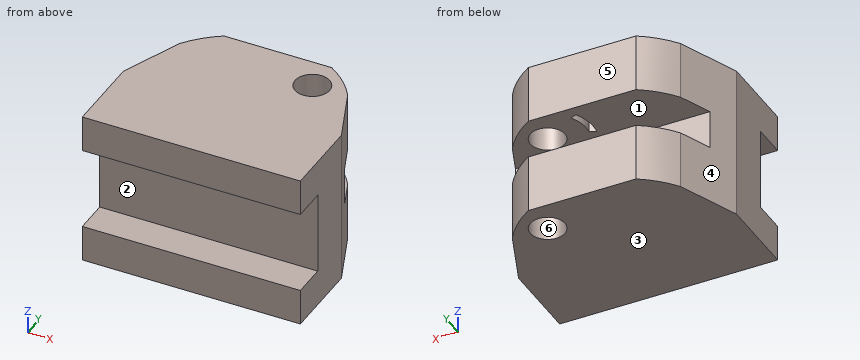
from build123d import *

# Parameters (mm, degrees)
SKETCH1_W           = 64
SKETCH1_H           = 33
BOSS_EXTRUDE2_DEPTH = 90
SKETCH5_W           = 34
SKETCH5_H           = 14
CUT_EXTRUDE1_DEPTH  = 91
SKETCH7_W           = 90
SKETCH7_H           = 64
BOSS_EXTRUDE3_DEPTH = 37
SKETCH9_W           = 16
SKETCH9_H           = 25
CUT_EXTRUDE2_DEPTH  = 91
CUT_EXTRUDE3_DEPTH  = 65
CUT_EXTRUDE4_DEPTH  = 65
SKETCH12_R          = 4.563258517
CUT_EXTRUDE5_DEPTH  = 65
SKETCH13_R          = 3.396180785
CUT_EXTRUDE7_DEPTH  = 4
SKETCH14_R          = 7.131807436
CUT_EXTRUDE8_DEPTH  = 65
CUT_EXTRUDE9_START  = -17
CUT_EXTRUDE9_DEPTH  = 30


with BuildPart() as part:
    # Sketch1 → Boss-Extrude2 (new body)
    with BuildSketch(Plane(origin=(0, 0, 0), x_dir=(0, 0, -1), z_dir=(1, 0, 0))):
        Rectangle(SKETCH1_W, SKETCH1_H)
    extrude(amount=BOSS_EXTRUDE2_DEPTH)

    # Sketch5 → Cut-Extrude1 (cut, through all)
    with BuildSketch(Plane.ZY):
        with Locations((0, -9.5)):
            Rectangle(SKETCH5_W, SKETCH5_H)
    extrude(amount=-CUT_EXTRUDE1_DEPTH, mode=Mode.SUBTRACT)

    # Sketch7 → Boss-Extrude3 (add)
    with BuildSketch(Plane(origin=(0, 16.5, 0), x_dir=(1, 0, 0), z_dir=(0, 1, 0))):
        with Locations((45, 0)):
            Rectangle(SKETCH7_W, SKETCH7_H)
    extrude(amount=BOSS_EXTRUDE3_DEPTH)

    # Sketch9 → Cut-Extrude2 (cut, through all)
    with BuildSketch(Plane.ZY):
        with Locations((0, 41)):
            Rectangle(SKETCH9_W, SKETCH9_H)
    extrude(amount=-CUT_EXTRUDE2_DEPTH, mode=Mode.SUBTRACT)

    # Sketch10 → Cut-Extrude3 (cut, through all)
    with BuildSketch(Plane.XY.offset(32)):
        Polygon((0, 16.5), (15, 53.5), (0, 53.5), align=None)
        Polygon((90, 53.5), (90, 16.5), (75, 53.5), align=None)
    extrude(amount=-CUT_EXTRUDE3_DEPTH, mode=Mode.SUBTRACT)

    # Sketch11 → Cut-Extrude4 (cut, through all)
    with BuildSketch(Plane.XY.offset(32)):
        with BuildLine():
            Line((22.559269827, 53.5), (15, 53.5))
            Line((15, 53.5), (10.196218084, 41.650671273))
            ThreePointArc((10.196218084, 41.650671273), (15.770987206, 48.208398087), (22.559269827, 53.5))
        make_face()
        with BuildLine():
            Line((80.252850536, 40.542968678), (75, 53.5))
            Line((75, 53.5), (66.982723611, 53.5))
            ThreePointArc((66.982723611, 53.5), (74.341930784, 47.763126364), (80.252850536, 40.542968678))
        make_face()
    extrude(amount=-CUT_EXTRUDE4_DEPTH, mode=Mode.SUBTRACT)

    # Sketch12 → Cut-Extrude5 (cut, through all)
    with BuildSketch(Plane(origin=(0, 0, -32), x_dir=(-1, 0, 0), z_dir=(0, 0, -1))):
        with Locations((-65.890311292, 40.12330388)):
            Circle(SKETCH12_R)
    extrude(amount=-CUT_EXTRUDE5_DEPTH, mode=Mode.SUBTRACT)

    # Sketch13 → Cut-Extrude7 (cut)
    with BuildSketch(Plane(origin=(0, 28.5, 0), x_dir=(1, 0, 0), z_dir=(0, 1, 0))):
        with Locations((18.559847102, 1.303256126)):
            Circle(SKETCH13_R)
    extrude(amount=-CUT_EXTRUDE7_DEPTH, mode=Mode.SUBTRACT)

    # Sketch14 → Cut-Extrude8 (cut, through all)
    with BuildSketch(Plane.XY.offset(32)):
        with Locations((65.890311292, 40.12330388)):
            Circle(SKETCH14_R)
    extrude(amount=-CUT_EXTRUDE8_DEPTH, mode=Mode.SUBTRACT)

    # Sketch15 → Cut-Extrude9 (cut)
    with BuildSketch(Plane.XY.offset(32).offset(CUT_EXTRUDE9_START)):
        with BuildLine():
            Line((52.144239181, 48.178611287), (49.568050992, 49.212876474))
            ThreePointArc((49.568050992, 49.212876474), (47.410527131, 42.86813331), (47.630804887, 36.170211787))
            Line((47.630804887, 36.170211787), (50.191024462, 37.407632885))
            ThreePointArc((50.191024462, 37.407632885), (50.21355191, 42.966135424), (52.144239181, 48.178611287))
        make_face()
    extrude(amount=-CUT_EXTRUDE9_DEPTH, mode=Mode.SUBTRACT)


solid = part.part
Can you work these out from the model? Positions are in its coordinate system, mm. Face numbers are marked on the shaded views. A direction names the side the tool comes from. Round coordinates to 2 decimals unless told otherwise and drop trailing zeros. Loops run counter-clockwise (first coordinate to the right, second up) from the corner with the lowest first, then second, coordinate; pieces in that order, holes last. Notation, with made-up numbers: (44, -4.5) - (69, -4.5) arc R17 cw to (69, 25.5) - close; hole circle Ø4 at (68, -30.5). An arc over 180 degrees is marked (long way). Write item = value, one per line. Start each with the question number.
(1) If we section it at A-A (y = -10.5): Please give me the cut outline in (x, z).
(2) If we section it at D-D (x = 63): Please give me the cut outline in (y, z), and give its area (3 significant figures).
(3) For the marked faces 1, 2 and 3, which set-ups out of +Z, -Z, +X, -X, +Y, -Y let a thin tool reach every point of the face, with its end or its side?
(4) If we mould it in two halves opening along X, with no side actions, what happens to the marked faces 4, 5 and 6? For each: released by +X, released by -X, zero draft, split by the parting line, or undercut.
(5) If I drill on probe 1 along Z at (x, y) = (81.5, -13); probe 2 along Y at (x, z) = (42.5, -0.5); probe 3 along Z at (x, y) = (45.5, 47), over which ranges is the centre line in solid material (lowest first)? Write a range as [from, to].
(6) If we section it at B-B (x = 54): Please give me the cut outline in (y, z).
(7) For P1, Ø4, axis at x = 54.5, z = -3.5, coming from the -Y side; P2, Ø7.5, axis at x = 17, z = 0, coming from the +Y side; P3, Ø13, axis at x = 65.89, y = 40.12, coming from the -Z side; P4, Ø4, axis at x = 18.56, z = -1.3, coming from the +Y side, each with a flat end and sliding along its axis, tell me the tip position at first contact or that it passes through.
(8) If we section it at C-C (z = -18.5): Please give me the cut outline in (x, y).
Ans:
q1.outline = (0, -32) - (90, -32) - (90, -17) - (0, -17) - close; (0, 17) - (90, 17) - (90, 32) - (0, 32) - close
q2.outline = (-16.5, -32) - (33.6, -32) - (33.6, -8) - (28.5, -8) - (28.5, 8) - (33.6, 8) - (33.6, 32) - (-16.5, 32) - (-16.5, 17) - (-2.5, 17) - (-2.5, -17) - (-16.5, -17) - close; (46.64, -32) - (53.5, -32) - (53.5, -8) - (46.64, -8) - close; (46.64, 8) - (53.5, 8) - (53.5, 32) - (46.64, 32) - close
q2.area = 2,980 mm²
q3.face_1 = +X, -X, +Y
q3.face_2 = +X, -X, -Y
q3.face_3 = -Z, +X, -X, +Y, -Y
q4.face_4 = released by -X
q4.face_5 = zero draft
q4.face_6 = undercut
q5.probe_1 = [-32, -17], [17, 32]
q5.probe_2 = [-2.5, 28.5]
q5.probe_3 = [-32, -8], [8, 32]
q6.outline = (-16.5, -32) - (53.5, -32) - (53.5, -8) - (28.5, -8) - (28.5, 8) - (53.5, 8) - (53.5, 32) - (-16.5, 32) - (-16.5, 17) - (-2.5, 17) - (-2.5, -17) - (-16.5, -17) - close
q7.P1 = -2.5
q7.P2 = 28.5
q7.P3 = through
q7.P4 = 24.5
q8.outline = (0, -16.5) - (90, -16.5) - (90, 16.5) - (80.25, 40.54) arc R42 ccw to (66.98, 53.5) - (22.56, 53.5) arc R42.24 ccw to (10.2, 41.65) - (0, 16.5) - close; hole circle Ø14.26 at (65.89, 40.12)
